from build123d import *

# Parameters (mm, degrees)
SKETCH1_W           = 812.8
SKETCH1_H           = 19.05
SKETCH1_W_2         = 19.05
BOSS_EXTRUDE2_DEPTH = 127
SKETCH2_R           = 3.81
CUT_EXTRUDE1_DEPTH  = 19.05
SKETCH3_R           = 19.05
CUT_EXTRUDE2_DEPTH  = 19.05
BOSS_EXTRUDE3_DEPTH = 13.97
SKETCH5_R           = 1.27
CUT_EXTRUDE3_DEPTH  = 19.05


with BuildPart() as part:
    # Sketch1 → Boss-Extrude2 (new body)
    with BuildSketch(Plane(origin=(0, 0, 0), x_dir=(1, 0, 0), z_dir=(0, 1, 0))):
        with Locations((406.4, -9.525)):
            Rectangle(SKETCH1_W, SKETCH1_H)
        with Locations((822.325, -9.525)):
            Rectangle(SKETCH1_W_2, SKETCH1_H)
        with Locations((-9.525, -9.525)):
            Rectangle(SKETCH1_W_2, SKETCH1_H)
    extrude(amount=BOSS_EXTRUDE2_DEPTH)

    # Sketch2 → Cut-Extrude1 (cut)
    with BuildSketch(Plane(origin=(0, 0, 0), x_dir=(-1, 0, 0), z_dir=(0, 0, -1))):
        with Locations((-14.224, 107.95)):
            Circle(SKETCH2_R)
        with Locations((-14.224, 63.5)):
            Circle(SKETCH2_R)
        with Locations((-14.224, 19.05)):
            Circle(SKETCH2_R)
        with Locations((-798.576, 19.05)):
            Circle(SKETCH2_R)
        with Locations((-798.576, 107.95)):
            Circle(SKETCH2_R)
        with Locations((-798.576, 63.5)):
            Circle(SKETCH2_R)
    extrude(amount=-CUT_EXTRUDE1_DEPTH, mode=Mode.SUBTRACT)

    # Sketch3 → Cut-Extrude2 (cut)
    with BuildSketch(Plane(origin=(0, 0, 0), x_dir=(-1, 0, 0), z_dir=(0, 0, -1))):
        with BuildLine():
            ThreePointArc((-663.448, 28.702), (-682.498, 9.652), (-701.548, 28.702))
            Line((-701.548, 28.702), (-701.548, 0))
            Line((-701.548, 0), (-663.448, 0))
            Line((-663.448, 0), (-663.448, 28.702))
        make_face()
        with Locations((-682.498, 28.702)):
            Circle(SKETCH3_R)
        with Locations((-406.4, 28.702)):
            Circle(SKETCH3_R)
        with BuildLine():
            Line((-425.45, 28.702), (-425.45, 0))
            Line((-425.45, 0), (-387.35, 0))
            Line((-387.35, 0), (-387.35, 28.702))
            ThreePointArc((-387.35, 28.702), (-406.4, 9.652), (-425.45, 28.702))
        make_face()
        with BuildLine():
            Line((-149.352, 28.702), (-149.352, 0))
            Line((-149.352, 0), (-111.252, 0))
            Line((-111.252, 0), (-111.252, 28.702))
            ThreePointArc((-111.252, 28.702), (-130.302, 9.652), (-149.352, 28.702))
        make_face()
        with Locations((-130.302, 28.702)):
            Circle(SKETCH3_R)
    extrude(amount=-CUT_EXTRUDE2_DEPTH, mode=Mode.SUBTRACT)

    # Sketch4 → Boss-Extrude3 (add)
    with BuildSketch(Plane(origin=(0, 0, 0), x_dir=(-1, 0, 0), z_dir=(0, 0, -1))):
        with BuildLine():
            ThreePointArc((-387.35, 28.702), (-406.4, 9.652), (-425.45, 28.702))
            Line((-425.45, 28.702), (-425.45, 0))
            Line((-425.45, 0), (-387.35, 0))
            Line((-387.35, 0), (-387.35, 28.702))
        make_face()
        with BuildLine():
            ThreePointArc((-387.35, 28.702), (-406.4, 47.752), (-425.45, 28.702))
            ThreePointArc((-425.45, 28.702), (-406.4, 9.652), (-387.35, 28.702))
        make_face()
        with BuildLine():
            Line((-111.252, 0), (-111.252, 28.702))
            ThreePointArc((-111.252, 28.702), (-130.302, 9.652), (-149.352, 28.702))
            Line((-149.352, 28.702), (-149.352, 0))
            Line((-149.352, 0), (-111.252, 0))
        make_face()
        with BuildLine():
            ThreePointArc((-149.352, 28.702), (-130.302, 9.652), (-111.252, 28.702))
            ThreePointArc((-111.252, 28.702), (-130.302, 47.752), (-149.352, 28.702))
        make_face()
        with BuildLine():
            Line((-663.448, 0), (-663.448, 28.702))
            ThreePointArc((-663.448, 28.702), (-682.498, 9.652), (-701.548, 28.702))
            Line((-701.548, 28.702), (-701.548, 0))
            Line((-701.548, 0), (-663.448, 0))
        make_face()
        with BuildLine():
            ThreePointArc((-701.548, 28.702), (-682.498, 9.652), (-663.448, 28.702))
            ThreePointArc((-663.448, 28.702), (-682.498, 47.752), (-701.548, 28.702))
        make_face()
    extrude(amount=-BOSS_EXTRUDE3_DEPTH)

    # Sketch5 → Cut-Extrude3 (cut)
    with BuildSketch(Plane.XY.offset(19.05)):
        with Locations((254, 91.948)):
            Circle(SKETCH5_R)
        with Locations((279.4, 91.948)):
            Circle(SKETCH5_R)
        with Locations((533.4, 91.948)):
            Circle(SKETCH5_R)
        with Locations((558.8, 91.948)):
            Circle(SKETCH5_R)
    extrude(amount=-CUT_EXTRUDE3_DEPTH, mode=Mode.SUBTRACT)


solid = part.part
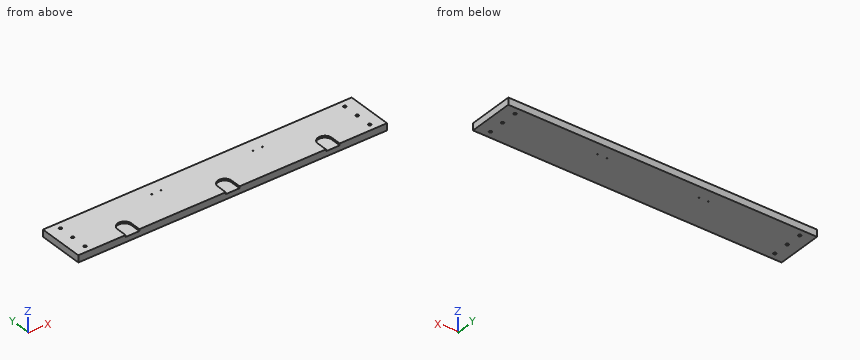
Read the model definition and answer for the solid it produces. Units are mm, in the model's axes. Round coordinates to 2 decimals unless told otherwise and drop trailing zeros. Order: outer loops, then holes, each group sorted by start corner. A loop starts at its lowest first (then second) coordinate and runs counter-clockwise, first axis right, second up.
1) The part is cut by section B-B on x = 118.5. Write down the section's boundary in (y, z), plus the area to 3 significant figures.
2) Straight lines are drawn through the part: L1, parallel to X at y = 19, z = 16.25; L2, parallel to Y at x = 533.4, z = 13.5; L3, parallel to Z at x = 689.5, y = 31. For each, find the intervals that lie inside material, in ascending order.
3) The part is cut by section A-A on x = 406.4. Write down the section's boundary in (y, z), plus the area to 3 significant figures.
4) Flat-ended cylindrical pins translate along their axes: pin 1 (8 mm diameter, centred on x = 719.5, z = 5.5, fed in from -Y); pin 2 (19 mm diameter, centred on x = 407.5, y = 27, fed in from +Z); pin 3 (2 mm diameter, centred on x = 558.8, y = 91.948, fed in from -Z). Find the tip coordinate at first contact, or state that the pin passes through.
Resolved:
1. outline: (0, 0) - (127, 0) - (127, 19.05) - (43.66, 19.05) - (43.66, 13.97) - (0, 13.97) - close
1. area: 2,200 mm2
2. L1: x = -19.05 to 10.41, 18.03 to 111.25, 149.35 to 387.35, 425.45 to 663.45, 701.55 to 794.77, 802.39 to 831.85
2. L2: y = 0 to 90.68, 93.22 to 127
2. L3: z = 0 to 13.97
3. outline: (0, 0) - (127, 0) - (127, 19.05) - (47.75, 19.05) - (47.75, 13.97) - (0, 13.97) - close
3. area: 2,180 mm2
4. pin 1: stops at y = 0
4. pin 2: stops at z = 13.97
4. pin 3: passes through
